Part model, mm, in its own coordinate system. Face numbers are marked on the shaded views. A direction names the side the tool comes from. Coordinates: 2 decimals unless noted, no trailing zeros. Order: outer loops, then holes, each group sorted by start corner. A loop starts at its lowest first (then second) coordinate and runs counter-clockwise, first axis right, second up.
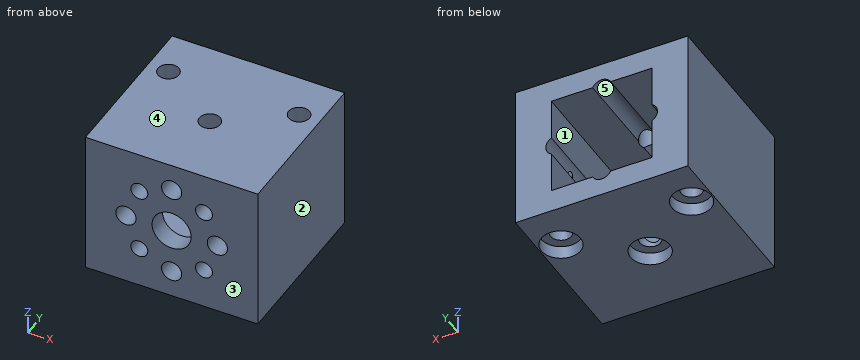
```python
from build123d import *

# Parameters (mm, degrees)
SKETCH_1_W          = 15.4
SKETCH_1_H          = 22.4
EXTRUDE_2_DEPTH     = 3
EXTRUDE_3_DEPTH     = 10
EXTRUDE_3_2_DEPTH   = 10
EXTRUDE_4_DEPTH     = 25
SKETCH_3_R          = 1.6
CUT_EXTRUDE_2_DEPTH = 31.8
SKETCH_9_R          = 1.3
SKETCH_9_R_2        = 3
SKETCH_9_R_3        = 1.55
CUT_EXTRUDE_6_DEPTH = 26
SKETCH_10_R         = 3
CUT_EXTRUDE_7_DEPTH = 2


with BuildPart() as part:
    # Sketch 1 → Extrude 2 (new body)
    with BuildSketch(Plane(origin=(0, 0, 0), x_dir=(1, 0, 0), z_dir=(0, 1, 0))):
        Rectangle(SKETCH_1_W, SKETCH_1_H)
    extrude(amount=EXTRUDE_2_DEPTH)



with BuildPart() as body_2:
    # Sketch 1_4 → Extrude 3 (new body)
    with BuildSketch(Plane(origin=(0, 0, 0), x_dir=(1, 0, 0), z_dir=(0, 1, 0))):
        Polygon((7.7, -11.2), (7.7, -7.7), (0, -7.7), (-4.7, -7.7), (-7.7, -7.7), (-7.7, -11.2), align=None)
    extrude(amount=EXTRUDE_3_DEPTH)


with BuildPart() as body_3:
    # Sketch 1_4 → Extrude 3 2 (new body)
    with BuildSketch(Plane(origin=(0, 0, 0), x_dir=(1, 0, 0), z_dir=(0, 1, 0))):
        Polygon((-7.7, 7.7), (0, 7.7), (7.7, 7.7), (7.7, 11.2), (-7.7, 11.2), align=None)
    extrude(amount=EXTRUDE_3_2_DEPTH)


with BuildPart() as part_1:
    add(part.part)

    add(body_2.part)  # Extrude 4 merges body 2

    add(body_3.part)  # Extrude 4 merges body 3
    # Sketch 1_5 → Extrude 4 (add)
    with BuildSketch(Plane(origin=(0, 0, 0), x_dir=(1, 0, 0), z_dir=(0, 1, 0))):
        Polygon((-7.7, 0), (-7.7, 7.7), (-7.7, 11.2), (-13.2, 11.2), (-13.2, -11.2), (-7.7, -11.2), (-7.7, -7.7), align=None)
        Polygon((7.7, 11.2), (7.7, 7.7), (7.7, 0), (7.7, -7.7), (7.7, -11.2), (13.2, -11.2), (13.2, 11.2), align=None)
        Polygon((7.7, -11.2), (7.7, -7.7), (0, -7.7), (-4.7, -7.7), (-7.7, -7.7), (-7.7, -11.2), align=None)
        Polygon((-7.7, 7.7), (0, 7.7), (7.7, 7.7), (7.7, 11.2), (-7.7, 11.2), align=None)
    extrude(amount=EXTRUDE_4_DEPTH)

    # Sketch 3 → Cut-Extrude 2 (cut, through all)
    with BuildSketch(Plane(origin=(0, 0, -19.6), x_dir=(-1, 0, 0), z_dir=(0, 0, -1))):
        with Locations((0, 11)):
            Circle(SKETCH_3_R)
        with Locations((-10, 17.91)):
            Circle(SKETCH_3_R)
        with Locations((10, 17.91)):
            Circle(SKETCH_3_R)
    extrude(amount=-CUT_EXTRUDE_2_DEPTH, mode=Mode.SUBTRACT)

    # Sketch 9 → Cut-Extrude 6 (cut, through all)
    with BuildSketch(Plane.XZ):
        with Locations((-4.949747468, -4.949747468)):
            Circle(SKETCH_9_R)
        with Locations((4.949747468, -4.949747468)):
            Circle(SKETCH_9_R)
        with Locations((4.949747468, 4.949747468)):
            Circle(SKETCH_9_R)
        with Locations((-4.949747468, 4.949747468)):
            Circle(SKETCH_9_R)
        Circle(SKETCH_9_R_2)
        with Locations((7, 0)):
            Circle(SKETCH_9_R_3)
        with Locations((0, 7)):
            Circle(SKETCH_9_R_3)
        with Locations((0, -7)):
            Circle(SKETCH_9_R_3)
        with Locations((-7, 0)):
            Circle(SKETCH_9_R_3)
    extrude(amount=-CUT_EXTRUDE_6_DEPTH, mode=Mode.SUBTRACT)

    # Sketch 10 → Cut-Extrude 7 (cut)
    with BuildSketch(Plane(origin=(0, 0, -11.2), x_dir=(-1, 0, 0), z_dir=(0, 0, -1))):
        with Locations((10, 17.91)):
            Circle(SKETCH_10_R)
        with Locations((0, 11)):
            Circle(SKETCH_10_R)
        with Locations((-10, 17.91)):
            Circle(SKETCH_10_R)
    extrude(amount=-CUT_EXTRUDE_7_DEPTH, mode=Mode.SUBTRACT)


solid = part_1.part
```
(1) Probe line 1 (Y direction, x = 10, z = -2); line 2 (Z direction, x = 3, y = 7.25); line 3 (X direction, y = 9.75, z = 0). List the from-to ranges inside material, lowest first.
(2) Slice it at A-A, the plane z = -7. Give the cut face in (x, y).
(3) Pull direction Z, two halves, no side cores. Call the marked faces 3, 4 and 5: +Z half, -Z half, draft (parallel to the pull), parting line (faces both ways), or undercut.
(4) Slice it at C-C, the plane y = 11. Give the cut face in (x, z).
(5) Slice it at D-D, the plane x = 10. Give the cut face in (y, z), then the cut area to 3 significant figures.
(6) Slice it at B-B, the plane x = 0. Give the cut face in (y, z), then the cut area to 3 significant figures.
(7) Drop flat-ended pins along their axis: pin 1 (7.5 mm diameter, centred on x = -2, z = 3, fed in from +Y); pin 2 (1.6 mm diameter, centred on x = 4.95, z = -4.95, fed in from +Y); pin 3 (1.8 mm diameter, centred on x = -9.5, y = 16.5, fed in from -Z). Give the stop position or say it passes through.
(8) Tool access for the marked faces 1 and 2: list every direction of +Z, -Z, +X, -X, +Y, -Y with a clear straight run to the whole face (end or side of a thin tool).
Here are the results:
1. line 1: y = 0 to 16.31, 19.51 to 25
1. line 2: z = -11.2 to -7.7, 7.7 to 11.2
1. line 3: x = -13.2 to -8.55, 8.55 to 13.2
2. outline: (-13.2, 0) - (-1.55, 0) - (-1.55, 3) - (-7.7, 3) - (-7.7, 25) - (-13.2, 25) - close; (1.55, 0) - (13.2, 0) - (13.2, 25) - (7.7, 25) - (7.7, 3) - (1.55, 3) - close; hole circle Ø3.2 at (-10, 17.91); hole circle Ø3.2 at (10, 17.91)
3. face 3: draft
3. face 4: +Z half
3. face 5: undercut
4. outline: (-13.2, -11.2) - (-3, -11.2) - (-3, -9.2) - (-1.6, -9.2) - (-1.6, -7.7) - (-7.7, -7.7) - (-7.7, -1.38) arc R1.55 cw to (-7.7, 1.38) - (-7.7, 7.7) - (-1.6, 7.7) - (-1.6, 11.2) - (-13.2, 11.2) - close; (1.6, -9.2) - (3, -9.2) - (3, -11.2) - (13.2, -11.2) - (13.2, 11.2) - (1.6, 11.2) - (1.6, 7.7) - (7.7, 7.7) - (7.7, 1.38) arc R1.55 cw to (7.7, -1.38) - (7.7, -7.7) - (1.6, -7.7) - close
5. outline: (0, -11.2) - (14.91, -11.2) - (14.91, -9.2) - (16.31, -9.2) - (16.31, 11.2) - (0, 11.2) - close; (19.51, -9.2) - (20.91, -9.2) - (20.91, -11.2) - (25, -11.2) - (25, 11.2) - (19.51, 11.2) - close
5. area: 483 mm2
6. outline: (0, -11.2) - (8, -11.2) - (8, -9.2) - (9.4, -9.2) - (9.4, -8.55) - (0, -8.55) - close; (0, -5.45) - (3, -5.45) - (3, -3) - (0, -3) - close; (0, 3) - (3, 3) - (3, 5.45) - (0, 5.45) - close; (0, 8.55) - (9.4, 8.55) - (9.4, 11.2) - (0, 11.2) - close; (12.6, -9.2) - (14, -9.2) - (14, -11.2) - (25, -11.2) - (25, -8.55) - (12.6, -8.55) - close; (12.6, 8.55) - (25, 8.55) - (25, 11.2) - (12.6, 11.2) - close
6. area: 125 mm2
7. pin 1: stops at y = 3
7. pin 2: passes through
7. pin 3: stops at z = -9.2
8. face 1: +Y
8. face 2: +Z, -Z, +X, +Y, -Y
